For this review, take the finished solid that the model builds, in its own axes (mm). Give positions to 0.01 mm unless a question says otherwise; leave off trailing zeros. Write each loop counter-clockwise with the first axis right and the second up, starting at its lowest first coordinate (ties: lowest second). Pieces come first, ordered by that corner, then holes.
Q1. For line 1 (Y direction, x = 0, z = -1.4); line 2 (Y direction, x = -6.25, z = 1.5); line 3 (Y direction, x = 6, z = 1.35), list the stretches that pass through material, from the lowest coordinate up.
Q2. Insertion check: P1, Ø1.4, axis at y = 12, z = -1, coming from the -X side; P2, Ø1.4, axis at x = 11.5, z = 0.5, coming from the +Y side; P3, Ø1.9, axis at y = 10.5, z = -0.5, coming from the +X side; P4, Ø1, axis at x = 1.5, y = 6.5, coming from the -Z side. Each pin has a flat end and moves straight along its axis. Give the tip position at first contact, or say it passes through.
Q3. We need section B-B (y = -4.5). Write out the cut boundary in (x, z), then the cut area to 3 significant figures.
Q4. We need section A-A (x = 10.5). Write out the cut boundary in (y, z).
Autodesk Inventor part; units mm, degrees
ref_plane "YZ Plane" through (0, 0, 0) normal (1, 0, 0) x (0, 1, 0)
ref_plane "XZ Plane" through (0, 0, 0) normal (0, 1, 0) x (-1, 0, 0)
ref_plane "XY Plane" through (0, 0, 0) normal (0, 0, 1) x (1, 0, 0)
sketch "Sketch1" plane through (0, 0, 0) normal (0, 0, 1) x (1, 0, 0)
  circle A0 centre (0, 0) radius 10
  circle A1 centre (0, 0) radius 12.5
  circle A2 centre (0, 0) radius 7.5
  line L0 (10, 0) -> (12.5, 0)
  line L1 (12.5, 0) -> (12.5, 1.75)
  line L2 (12.5, 1.75) -> (10, 1.75)
  line L3 (10, 1.75) -> (10, 0)
  line L4 (12.5, 0) -> (12.5, -1.75)
  line L5 (12.5, -1.75) -> (10, -1.75)
  line L6 (10, -1.75) -> (10, 0)
  line L7 (10.0763, 7.6014) -> (8.3085, 5.8336)
  line L8 (8.3085, 5.8336) -> (7.0711, 7.0711)
  line L9 (5.8336, 8.3085) -> (7.0711, 7.0711)
  line L10 (7.6014, 10.0763) -> (5.8336, 8.3085)
  line L11 (8.8388, 8.8388) -> (7.6014, 10.0763)
  line L12 (8.8388, 8.8388) -> (10.0763, 7.6014)
  line L13 (1.75, 12.5) -> (1.75, 10)
  line L14 (1.75, 10) -> (0, 10)
  line L15 (-1.75, 10) -> (0, 10)
  line L16 (-1.75, 12.5) -> (-1.75, 10)
  line L17 (0, 12.5) -> (-1.75, 12.5)
  line L18 (0, 12.5) -> (1.75, 12.5)
  line L19 (-7.6014, 10.0763) -> (-5.8336, 8.3085)
  line L20 (-5.8336, 8.3085) -> (-7.0711, 7.0711)
  line L21 (-8.3085, 5.8336) -> (-7.0711, 7.0711)
  line L22 (-10.0763, 7.6014) -> (-8.3085, 5.8336)
  line L23 (-8.8388, 8.8388) -> (-10.0763, 7.6014)
  line L24 (-8.8388, 8.8388) -> (-7.6014, 10.0763)
  line L25 (-12.5, 1.75) -> (-10, 1.75)
  line L26 (-10, 1.75) -> (-10, 0)
  line L27 (-10, -1.75) -> (-10, 0)
  line L28 (-12.5, -1.75) -> (-10, -1.75)
  line L29 (-12.5, 0) -> (-12.5, -1.75)
  line L30 (-12.5, 0) -> (-12.5, 1.75)
  line L31 (-10.0763, -7.6014) -> (-8.3085, -5.8336)
  line L32 (-8.3085, -5.8336) -> (-7.0711, -7.0711)
  line L33 (-5.8336, -8.3085) -> (-7.0711, -7.0711)
  line L34 (-7.6014, -10.0763) -> (-5.8336, -8.3085)
  line L35 (-8.8388, -8.8388) -> (-7.6014, -10.0763)
  line L36 (-8.8388, -8.8388) -> (-10.0763, -7.6014)
  line L37 (-1.75, -12.5) -> (-1.75, -10)
  line L38 (-1.75, -10) -> (0, -10)
  line L39 (1.75, -10) -> (0, -10)
  line L40 (1.75, -12.5) -> (1.75, -10)
  line L41 (0, -12.5) -> (1.75, -12.5)
  line L42 (0, -12.5) -> (-1.75, -12.5)
  line L43 (7.6014, -10.0763) -> (5.8336, -8.3085)
  line L44 (5.8336, -8.3085) -> (7.0711, -7.0711)
  line L45 (8.3085, -5.8336) -> (7.0711, -7.0711)
  line L46 (10.0763, -7.6014) -> (8.3085, -5.8336)
  line L47 (8.8388, -8.8388) -> (10.0763, -7.6014)
  line L48 (8.8388, -8.8388) -> (7.6014, -10.0763)
  point P0 (-1.75, 12.3769)
  point P1 (-7.5143, 9.9892)
  point P2 (-9.9892, 7.5143)
  point P3 (-12.3769, 1.75)
  point P4 (-12.3769, -1.75)
  point P5 (-9.9892, -7.5143)
  point P6 (-7.5143, -9.9892)
  point P7 (-1.75, -12.3769)
  point P8 (1.75, -12.3769)
  point P9 (7.5143, -9.9892)
  point P10 (9.9892, -7.5143)
  point P11 (12.3769, -1.75)
  point P12 (12.3769, 1.75)
  point P13 (9.9892, 7.5143)
  point P14 (7.5143, 9.9892)
  point P15 (1.75, 12.3769)
  dimension "d10" = 20
  dimension "d11" = 2.5
  dimension "d12" = 2.5
  dimension "d13" = 1.75
  dimension "d16" = 360
extrude "Extrusion1" add sketch "Sketch1" along normal mid plane 3.5 contours A0 | L6 L5 A1 L46 L45 A0 | A0 L8 L7 A1 L2 L3 | A0 L14 L13 A1 L10 L9 | L44 L43 A1 L40 L39 A0 | A0 L20 L19 A1 L16 L15 | L38 L37 A1 L34 L33 A0 | A0 L26 L25 A1 L22 L21 | L32 L31 A1 L28 L27 A0
properties part number "Vrhnji obrok"
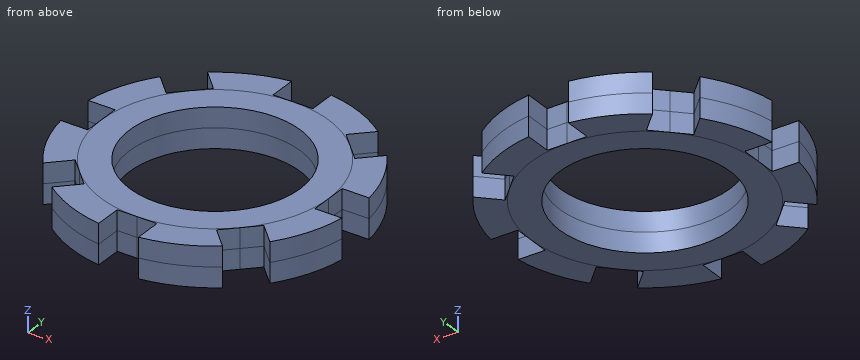
Computed:
1. line 1: y = -10 to -7.5, 7.5 to 10
1. line 2: y = -10.83 to -8.72, -7.89 to -4.15, 4.15 to 7.89, 8.72 to 10.83
1. line 3: y = -10.97 to -8.47, -8.14 to -4.5, 4.5 to 8.14, 8.47 to 10.97
2. P1: stops at x = -5.34
2. P2: stops at y = 6.29
2. P3: stops at x = 7.51
2. P4: passes through
3. outline: (-11.66, -1.75) - (-6, -1.75) - (-6, 1.75) - (-11.66, 1.75) - close; (6, -1.75) - (11.66, -1.75) - (11.66, 1.75) - (6, 1.75) - close
3. area: 39.6 mm2
4. outline: (-6.78, -1.75) - (-1.75, -1.75) - (-1.75, 1.75) - (-6.78, 1.75) - close; (1.75, -1.75) - (6.78, -1.75) - (6.78, 1.75) - (1.75, 1.75) - close
